Geometry: see drawing. Coordinates: mm, zero at the bounding-box minimum. Give positions to 0.01 mm unless a question says otherwise; leave off trailing zeros. Loops run counter-clockwise (first coordinate to the right, second up) from the corner with the lowest first, then second, coordinate; pieces in that order, holes last. Notation, with made-up numbers: M -28.75,67.5 L 7.25,67.5 A8 cw 7.25,72.5 Z; hole C 4.25,-32.75 d5. An arc over 180 degrees is marked long. Answer in a Markdown table with one row per item.
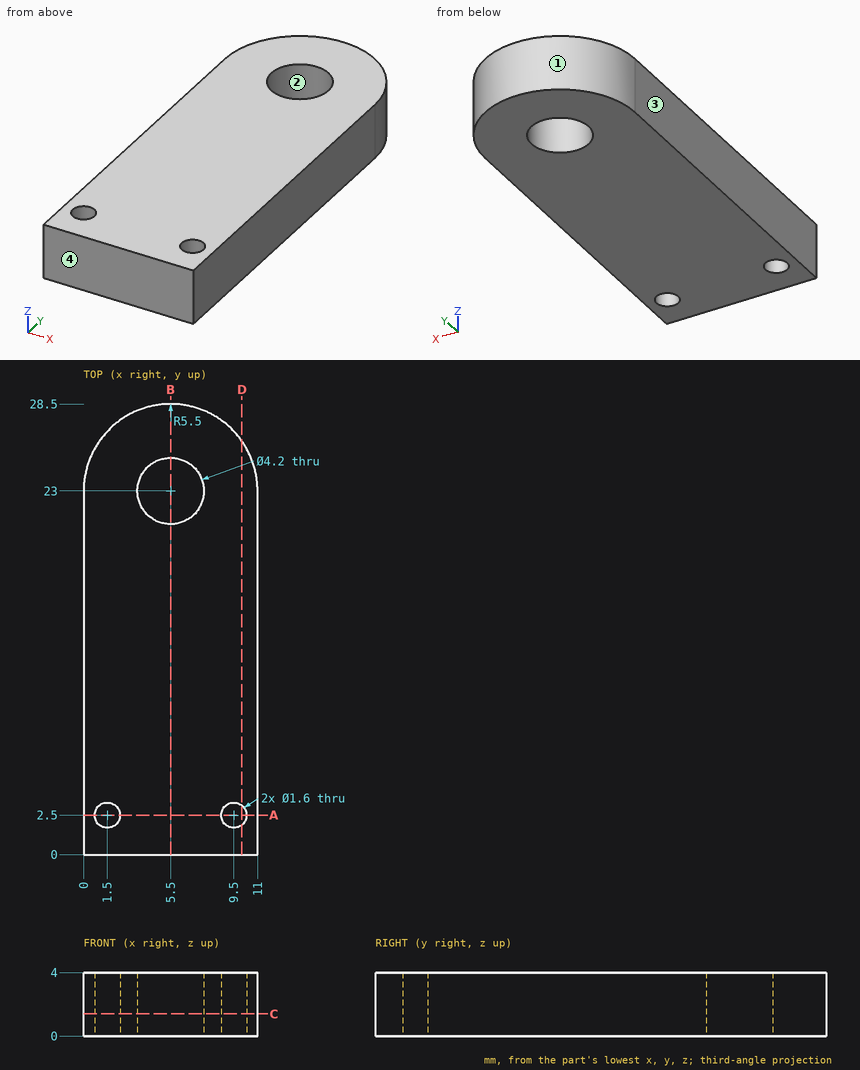
1) Section B-B, the plane x = 5.5. Return loops of the section in (y, z), then the cut area to 3 significant figures.
Reply:
| item | result |
|---|---|
| outline | M 0,0 L 20.9,0 L 20.9,4 L 0,4 Z; M 25.1,0 L 28.5,0 L 28.5,4 L 25.1,4 Z |
| area | 97.2 mm² |
2) Section A-A, the plane y = 2.5. Return loops of the section in (x, z), then the cut area to 3 significant figures.
Reply:
| item | result |
|---|---|
| outline | M 0,0 L 0.7,0 L 0.7,4 L 0,4 Z; M 2.3,0 L 8.7,0 L 8.7,4 L 2.3,4 Z; M 10.3,0 L 11,0 L 11,4 L 10.3,4 Z |
| area | 31.2 mm² |
3) Pull-direction query (Y, two-part tool) for the marked faces 1, 2, 3 and 4; classes: released by +Y, released by -Y, zero draft, split by the parting line, or undercut.
Reply:
| item | result |
|---|---|
| face 1 | released by +Y |
| face 2 | undercut |
| face 3 | zero draft |
| face 4 | released by -Y |
4) Material intervals for L1, parallel to Y at x = 5.5, z = 1.25; L2, parallel to X at y = 2.75, z = 3.45; L3, parallel to Y at x = 9.5, z = 1.85, sorted ascending.
Reply:
| item | result |
|---|---|
| L1 | y = 0 to 20.9, 25.1 to 28.5 |
| L2 | x = 0 to 0.74, 2.26 to 8.74, 10.26 to 11 |
| L3 | y = 0 to 1.7, 3.3 to 26.77 |
5) Pin query (flat end, axial travel): pin 1 Ø1 at (x, y) = (1.5, 2.5) entering from +Z. Return the tip coordinate at first contact, or that it passes through.
Reply:
| item | result |
|---|---|
| pin 1 | passes through |
6) Section C-C, the plane z = 1.4. Return loops of the section in (x, y), then the cut area to 3 significant figures.
Reply:
| item | result |
|---|---|
| outline | M 0,0 L 11,0 L 11,23 A5.5 ccw 0,23 Z; hole C 1.5,2.5 d1.6; hole C 5.5,23 d4.2; hole C 9.5,2.5 d1.6 |
| area | 283 mm² |
7) Section D-D, the plane x = 10. Return loops of the section in (y, z), then the cut area to 3 significant figures.
Reply:
| item | result |
|---|---|
| outline | M 0,0 L 1.88,0 L 1.88,4 L 0,4 Z; M 3.12,0 L 26.16,0 L 26.16,4 L 3.12,4 Z |
| area | 99.7 mm² |
